Input: part model. Units: mm. Frame: model coordinates. A direction names the side the tool comes from. Round coordinates to 2 decimals unless told otherwise and drop trailing zeros. Loops run counter-clockwise (first coordinate to the right, second up) from the corner with the lowest first, then second, coordinate; pieces in that order, holes last. Notation, with made-up numbers: M 88,41 L 117,41 A5 cw 117,46 Z; hole C 86.5,49.25 d7. An arc over 180 degrees is marked long. Put each result on its own line as item: value. Start each with the question number.
1) Section C-C on y = 12. Output: boundary loops of the cut face in (x, z).
2) Section D-D on z = 1. Output: boundary loops of the cut face in (x, y).
3) Draft query along X for faces 1 (the face through (0, 10, 1)), 2 (the face through (50, 0, 1)), 3 (the face through (-1, 1, 2.5)). Return one class per face: +X half, -X half, draft (parallel to the pull), parting line (faces both ways), or undercut.
4) Reachability of faces 4 (the face through (1, -25, 1)), 5 (the face through (35, 12, 1)), 6 (the face through (-0.7, 25.625, 1.232)) from +Z, -Z, +X, -X, +Y, -Y: full face, straight path, thin tool, end or side. Return the list, or none.
5) Line query: probe 1 along Y at (x, z) = (7, 0.95); probe 2 along Y at (x, z) = (25.25, 0.75); probe 3 along Y at (x, z) = (27, 1.65). Output: solid intervals per line, ascending.
6) Section A-A on y = 21. Output: boundary loops of the cut face in (x, z), plus the area to 3 significant figures.
7) Section B-B on x = 22. Output: boundary loops of the cut face in (y, z).
Autodesk Inventor part; units mm, degrees
ref_plane "YZ Plane" through (0, 0, 0) normal (1, 0, 0) x (0, 1, 0)
ref_plane "XZ Plane" through (0, 0, 0) normal (0, 1, 0) x (-1, 0, 0)
ref_plane "XY Plane" through (0, 0, 0) normal (0, 0, 1) x (1, 0, 0)
sketch "Sketch1" plane through (0, 0, 0) normal (0, 0, 1) x (1, 0, 0)
  line L0 (-50, 25) -> (50, 25)
  line L1 (50, 25) -> (50, -25)
  line L2 (50, -25) -> (-50, -25)
  line L3 (-50, -25) -> (-50, 25)
  line L4 (-35, 12) -> (35, 12) construction
  line L5 (-33, 10) -> (33, 10)
  line L6 (33, 14) -> (-33, 14)
  arc A0 (-33, 14) -> (-33, 10) centre (-33, 12) ccw
  arc A1 (33, 10) -> (33, 14) centre (33, 12) ccw
  arc A2 (50, 25) -> (-50, 25) centre (0, -1974.3749) ccw
  circle A3 centre (-25.25, 6) radius 1.5
  circle A4 centre (25.25, 6) radius 1.5
  circle A5 centre (-7, 21) radius 1.5
  circle A6 centre (7, 21) radius 1.5
  line L7 (0, 134.945) -> (0, -92.5364) construction
  point P0 (0, 0)
  point P1 (50, 0)
  point P2 (0, -25)
  point P3 (0, 12)
  point P4 (35, 25.3188)
  point P5 (35, 6)
  dimension "d0" = 50
  dimension "d1" = 100
  dimension "d2" = 4
  dimension "d4" = 66
  dimension "d5" = 2000
  dimension "d6" = 50.5
  dimension "d7" = 3
  dimension "d8" = 14
  dimension "d9" = 9
  dimension "d10" = 4
  dimension "d11" = 6
  dimension "d14" = 13.3188
  dimension "d15" = 19.3188
extrude "Extrusion1" add sketch "Sketch1" along normal blind 2.5
properties part number "platform_part"
Geometry results:
1. outline: M -50,0 L -35,0 L -35,2.5 L -50,2.5 Z; M 35,0 L 50,0 L 50,2.5 L 35,2.5 Z
2. outline: M -50,-25 L 50,-25 L 50,25 A2000 ccw -50,25 Z; hole M -33,10 L 33,10 A2 ccw 33,14 L -33,14 A2 ccw Z; hole C -25.25,6 d3; hole C -7,21 d3; hole C 7,21 d3; hole C 25.25,6 d3
3. face 1: undercut
3. face 2: +X half
3. face 3: draft
4. face 4: +Z, -Z, +X, -X, -Y
4. face 5: +Z, -Z
4. face 6: +Z, -Z, +Y
5. probe 1: y = -25 to 10, 14 to 19.5, 22.5 to 25.61
5. probe 2: y = -25 to 4.5, 7.5 to 10, 14 to 25.47
5. probe 3: y = -25 to 10, 14 to 25.44
6. outline: M -50,0 L -8.5,0 L -8.5,2.5 L -50,2.5 Z; M -5.5,0 L 5.5,0 L 5.5,2.5 L -5.5,2.5 Z; M 8.5,0 L 50,0 L 50,2.5 L 8.5,2.5 Z
6. area: 235 mm²
7. outline: M -25,0 L 10,0 L 10,2.5 L -25,2.5 Z; M 14,0 L 25.5,0 L 25.5,2.5 L 14,2.5 Z
